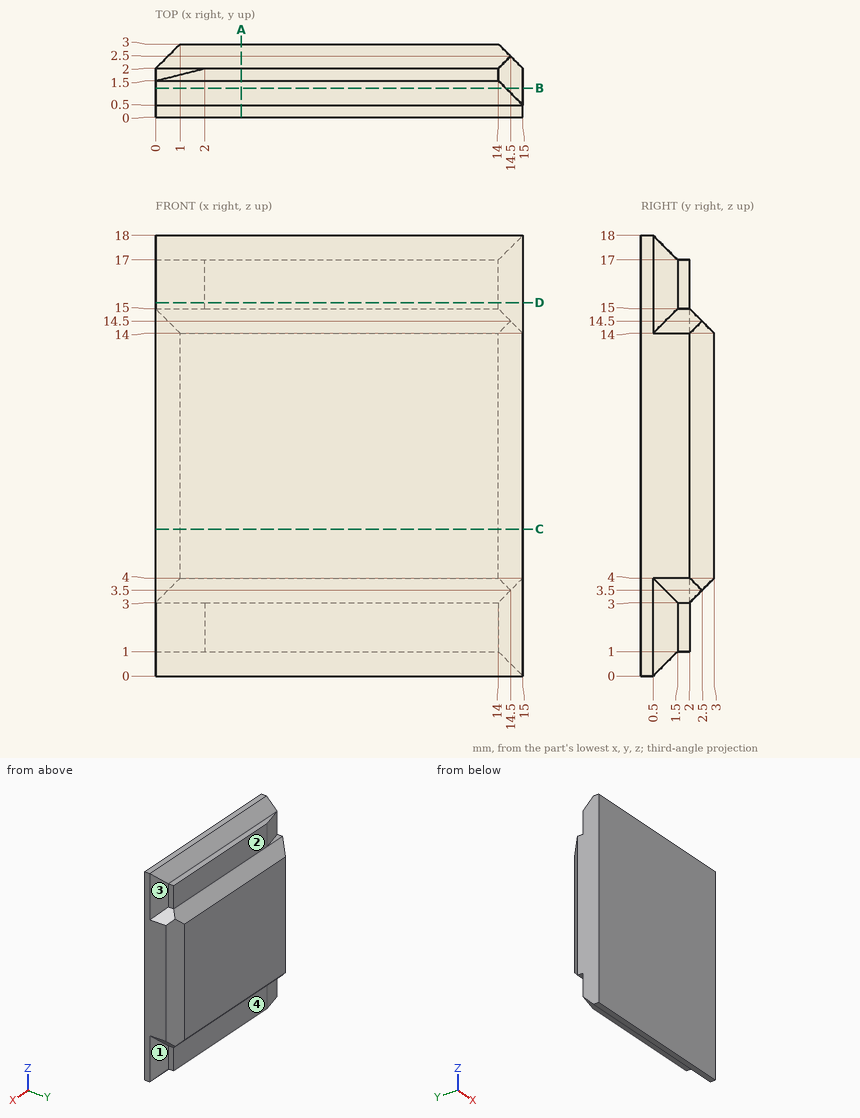
Answer from the drawing. Dimensions are ordinates in mm from the lowest x, y and z of the part. A direction names the side the tool comes from. Coordinates: 2 decimals unless noted, no trailing zeros. Write each loop counter-clockwise with the first axis right and the second up, starting at its lowest first coordinate (ties: lowest second). Pieces come first, ordered by that corner, then holes. Notation, with made-up numbers: M 50.25,15 L 72.25,15 A7 cw 72.25,25 Z; hole C -32,-18 d10. An arc over 180 degrees is marked long. Put each result on its own line as item: value. Start each with the question number.
1. A cutting plane is placed at B-B on y = 1.2. Write down the section's boundary in (x, z), then the cut area to 3 significant figures.
2. A cutting plane is placed at A-A on x = 3.5. Write down the section's boundary in (y, z), then the cut area to 3 significant figures.
3. Flat-ended cylindrical pins translate along their axes: P1, Ø1.6, axis at x = 7.5, z = 16, coming from the +Y side; P2, Ø3, axis at x = 4, z = 16, coming from the -Y side; P3, Ø1.6, axis at x = 5.5, z = 2.5, coming from the +Y side. Find the tip coordinate at first contact, or state that the pin passes through.
4. A cutting plane is placed at D-D on z = 15.25. Write down the section's boundary in (x, y).
5. Which of the six approach directions +Z, -Z, +X, -X, +Y, -Y give full straight-line access (tool end or side, diameter ignored) to the marked faces 1, 2, 3 and 4?
6. A cutting plane is placed at C-C on z = 6. Write down the section's boundary in (x, y), then the cut area to 3 significant figures.
7. Consider line 1 (Y direction, x = 12.25, z = 16); line 2 (Z direction, x = 14.5, y = 2.45); line 3 (X direction, y = 2.5, z = 12). Determine where each line is inside the solid, lowest interval first. Write a range as from..to.
Resolved:
1. outline: M 0,0.7 L 14.3,0.7 L 14.3,3.3 L 15,4 L 15,14 L 14.3,14.7 L 14.3,17.3 L 0,17.3 Z
1. area: 245 mm2
2. outline: M 0,0 L 0.5,0 L 1.5,1 L 2,1 L 2,3 L 3,4 L 3,14 L 2,15 L 2,17 L 1.5,17 L 0.5,18 L 0,18 Z
2. area: 45.0 mm2
3. P1: stops at y = 2
3. P2: stops at y = 0
3. P3: stops at y = 2.3
4. outline: M 0,0 L 15,0 L 15,0.5 L 14,1.5 L 14,2 L 2,2 L 0,1.5 Z
5. face 1: -Z, +X, +Y
5. face 2: +Z, +X, -X, +Y
5. face 3: +Z, +X, +Y
5. face 4: -Z, +X, -X, +Y
6. outline: M 0,0 L 15,0 L 15,2 L 14,3 L 1,3 L 0,2 Z
6. area: 44.0 mm2
7. line 1: y = 0..2
7. line 2: z = 3.5..14.5
7. line 3: x = 0.5..14.5
